The model under review builds one solid part; all positions refer to its coordinate system, in mm. Give positions to 0.01 mm unless a question says otherwise; leave off trailing zeros. Order: outer loops, then holes, each group sorted by start corner. A loop starts at its lowest first (then second) coordinate and runs counter-clockwise, first axis right, second up. Notation, with made-up numbers: (71.5, 16.25) -> (95.5, 16.25) arc R25 ccw to (95.5, 52.25) -> close; hole circle Ø7 at (84.5, 33). An arc over 180 degrees is marked (long way). Answer as a JSON object with one key per item and string values. Group by question number.
Autodesk Fusion 360 part; units mm, degrees
sketch "Sketch1" plane through (0, 0, 0) normal (0, 0, 1) x (1, 0, 0)
  circle A0 centre (0, 0) radius 34
  dimension "MotorDia" = 68
extrude "Extrude1" add sketch "Sketch1" along normal blind 33.8
chamfer "Chamfer1" distance 4 distance2 9 1 edges at (-31.6991, -12.2949, 0) measured on face at (33.9577, -1.6948, 22.5333)
chamfer "Chamfer2" distance 20 distance2 9 1 edges at (-31.6991, -12.2949, 33.8) measured on face at (10.8298, 6.4941, 33.8)
1. Take a section at C-C on z = 5. Give the boundary of the cut face in (x, y), plus the area to 3 significant figures.
2. For pin 1 (10 mm diameter, centred on x = 18, z = 19, fed in from +Y); pin 2 (2 mm diameter, centred on x = -26, y = 15.5, fed in from +Z); pin 3 (1.5 mm diameter, centred on y = -23.5, z = 13.5, fed in from +X), all flat-tipped, find the tip position at first contact; note any pin that passes through.
3. For probe 1 along Y at (x, z) = (-0.5, 17.5); probe 2 along X at (y, z) = (-17, 16); probe 3 along Y at (x, z) = (-9, 24), list the stretches that pass through material, from the lowest coordinate up. Write a range as [from, to].
4. Take a section at A-A on y = 0. Give the boundary of the cut face in (x, z).
Checks:
{
 "1": {"outline": "circle Ø68 at (0, 0)", "area": "3,630 mm2"},
 "2": {"pin 1": "stops at y = 31.42", "pin 2": "stops at z = 26.93", "pin 3": "stops at x = 25.27"},
 "3": {"probe 1": "y = [-34, 34]", "probe 2": "x = [-29.44, 29.44]", "probe 3": "y = [-32.79, 32.79]"},
 "4": {"outline": "(-34, 4) -> (-25, 0) -> (25, 0) -> (34, 4) -> (34, 24.8) -> (14, 33.8) -> (-14, 33.8) -> (-34, 24.8) -> close"}
}
